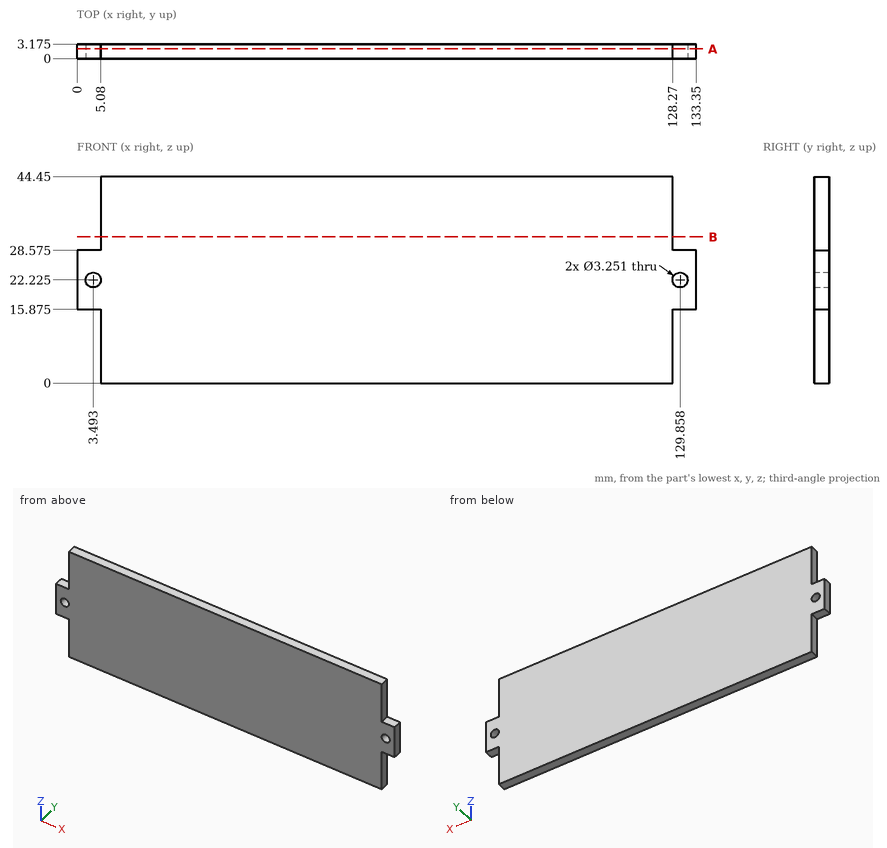
Verification items for this drawing (mm, ordinates from the low corner). Coordinates: 2 decimals unless noted, no trailing zeros. Order: outer loops, then holes, each group sorted by start corner. A loop starts at its lowest first (then second) coordinate and runs counter-clockwise, first axis right, second up. Notation, with made-up numbers: (79, -7.5) - (109, -7.5) arc R11 cw to (109, -2.5) - close; hole circle Ø5 at (38.25, 57). An arc over 180 degrees is marked (long way). Use one line per item in the form item = value.
1. Gauge pin test, flat ends, axial feed: pin 1 (1.6 mm diameter, centred on y = 2, z = 7.5, fed in from +X); pin 2 (1.6 mm diameter, centred on x = 3, y = 1, fed in from -Z) (1 decimal); pin 3 (3 mm diameter, centred on x = 129.86, z = 22.22, fed in from -Y); pin 4 (1.6 mm diameter, centred on y = 1.5, z = 37.5, fed in from -X). Record the tip position at first contact, or that the pin passes through.
Here are the results:
pin_1 = 128.27
pin_2 = 15.9
pin_3 = through
pin_4 = 5.08
2. Scan lines: line 1 (X direction, y = 1.65, z = 38); line 2 (X direction, y = 0.75, z = 21.5). Record each from-to range of solid material in increasing order.
Here are the results:
line_1 = 5.08 to 128.27
line_2 = 0 to 2.04, 4.95 to 128.4, 131.31 to 133.35
3. Section check B-B (z = 31.5). Record the boundary of the cut face in (x, y) (1 decimal), then the cut area to 3 significant figures.
Here are the results:
outline = (5.1, 0) - (128.3, 0) - (128.3, 3.2) - (5.1, 3.2) - close
area = 391 mm²
4. Section check A-A (y = 2.15). State how many separate pieces and enclosed holes the cut face has, then the cut area to 3 significant figures.
Here are the results:
separate_pieces = 1
enclosed_holes = 2
area = 5,590 mm²
